```python
from build123d import *

# Parameters (mm, degrees)
SKETCH1_R              = 6.35
SKETCH1_R_2            = 3.175
BOSS_EXTRUDE1_DEPTH    = 12.7
CUT_EXTRUDE1_DEPTH     = 10.795
CUT_EXTRUDE2_START     = -29
CUT_EXTRUDE2_OUTLINE_R = 1.905
CUT_EXTRUDE2_DEPTH     = 58
SKETCH3_R              = 8.128
SKETCH3_R_2            = 6.35
BOSS_EXTRUDE2_DEPTH    = 1.27
SKETCH4_R              = 1.5875
SKETCH4_R_2            = 1.143
CUT_EXTRUDE3_DEPTH     = 31.75
SKETCH5_R              = 1.905
CUT_EXTRUDE4_DEPTH     = 7.62
SKETCH6_W              = 3.175
SKETCH6_H              = 7.353822806
CUT_EXTRUDE5_DEPTH     = 1.016
SKETCH7_R              = 4.445
CUT_EXTRUDE6_DEPTH     = 1.27


with BuildPart() as part:
    # Sketch1 → Boss-Extrude1 (new body)
    with BuildSketch(Plane.XY):
        with BuildLine():
            Line((-15.875, 228.6), (-15.875, 41.885940063))
            ThreePointArc((-15.875, 41.885940063), (-17.859739298, 27.82498979), (-23.658870968, 14.862752926))
            ThreePointArc((-23.658870968, 14.862752926), (-27.242520167, -6.203925768), (-14.890307558, -23.641538462))
            Line((-14.890307558, -23.641538462), (-4.737825132, -30.035944056))
            ThreePointArc((-4.737825132, -30.035944056), (0, -31.403636364), (4.737825132, -30.035944056))
            Line((4.737825132, -30.035944056), (14.890307558, -23.641538462))
            ThreePointArc((14.890307558, -23.641538462), (27.242520167, -6.203925768), (23.658870968, 14.862752926))
            ThreePointArc((23.658870968, 14.862752926), (17.859739298, 27.82498979), (15.875, 41.885940063))
            Line((15.875, 41.885940063), (15.875, 228.6))
            ThreePointArc((15.875, 228.6), (0, 244.475), (-15.875, 228.6))
        make_face()
        Circle(SKETCH1_R, mode=Mode.SUBTRACT)
        with Locations((0, 228.6)):
            Circle(SKETCH1_R_2, mode=Mode.SUBTRACT)
    extrude(amount=BOSS_EXTRUDE1_DEPTH)

    # Sketch2 → Cut-Extrude1 (cut)
    with BuildSketch(Plane.XY.offset(12.7)):
        with BuildLine():
            Line((-11.43, 222.25), (11.43, 222.25))
            ThreePointArc((11.43, 222.25), (13.226051224, 221.506051224), (13.97, 219.71))
            Line((13.97, 219.71), (13.97, 21.969531743))
            ThreePointArc((13.97, 21.969531743), (0, -26.035), (-13.97, 21.969531743))
            Line((-13.97, 21.969531743), (-13.97, 219.71))
            ThreePointArc((-13.97, 219.71), (-13.226051224, 221.506051224), (-11.43, 222.25))
        make_face()
    extrude(amount=-CUT_EXTRUDE1_DEPTH, mode=Mode.SUBTRACT)

    # Cut-Extrude2: read off the stored shape, not the designer's step
    # Cut-Extrude2 outline → Cut-Extrude2 (cut)
    with BuildSketch(Plane.YZ.offset(CUT_EXTRUDE2_START)):
        with Locations((0, 6.985)):
            Circle(CUT_EXTRUDE2_OUTLINE_R)
    extrude(amount=CUT_EXTRUDE2_DEPTH, mode=Mode.SUBTRACT)

    # Sketch3 → Boss-Extrude2 (add)
    with BuildSketch(Plane.XY.offset(1.905)):
        Circle(SKETCH3_R)
        Circle(SKETCH3_R_2, mode=Mode.SUBTRACT)
    extrude(amount=BOSS_EXTRUDE2_DEPTH)

    # Sketch4 → Cut-Extrude3 (cut)
    with BuildSketch(Plane.XY.offset(12.7)):
        with Locations((0, 219.71)):
            Circle(SKETCH4_R)
        with Locations((-6.35, 184.15)):
            Circle(SKETCH4_R_2)
        with Locations((6.35, 184.15)):
            Circle(SKETCH4_R_2)
        with Locations((-6.35, 69.85)):
            Circle(SKETCH4_R_2)
        with Locations((6.35, 69.85)):
            Circle(SKETCH4_R_2)
        with Locations((-16.764, 23.241)):
            Circle(SKETCH4_R_2)
        with Locations((16.764, 23.241)):
            Circle(SKETCH4_R_2)
        with Locations((0, -28.575)):
            Circle(SKETCH4_R_2)
        with Locations((-10.4775, 28.1178)):
            Circle(SKETCH4_R_2)
        with Locations((10.4775, 28.1178)):
            Circle(SKETCH4_R_2)
    extrude(amount=-CUT_EXTRUDE3_DEPTH, mode=Mode.SUBTRACT)

    # Sketch5 → Cut-Extrude4 (cut)
    with BuildSketch(Plane.XY.offset(12.7)):
        with Locations((-11.43, 228.6)):
            Circle(SKETCH5_R)
        with Locations((-9.898670365, 234.315)):
            Circle(SKETCH5_R)
        with Locations((-5.715, 238.498670365)):
            Circle(SKETCH5_R)
        with Locations((0, 240.03)):
            Circle(SKETCH5_R)
        with Locations((5.715, 238.498670365)):
            Circle(SKETCH5_R)
        with Locations((9.898670365, 234.315)):
            Circle(SKETCH5_R)
        with Locations((11.43, 228.6)):
            Circle(SKETCH5_R)
    extrude(amount=-CUT_EXTRUDE4_DEPTH, mode=Mode.SUBTRACT)

    # Sketch6 → Cut-Extrude5 (cut)
    with BuildSketch(Plane(origin=(0, 0, 0), x_dir=(-1, 0, 0), z_dir=(0, 0, -1))):
        with Locations((0, 223.386911403)):
            Rectangle(SKETCH6_W, SKETCH6_H)
    extrude(amount=-CUT_EXTRUDE5_DEPTH, mode=Mode.SUBTRACT)

    # Sketch7 → Cut-Extrude6 (cut)
    with BuildSketch(Plane(origin=(0, 0, 0), x_dir=(-1, 0, 0), z_dir=(0, 0, -1))):
        with Locations((0, 228.6)):
            Circle(SKETCH7_R)
    extrude(amount=-CUT_EXTRUDE6_DEPTH, mode=Mode.SUBTRACT)


solid = part.part
```
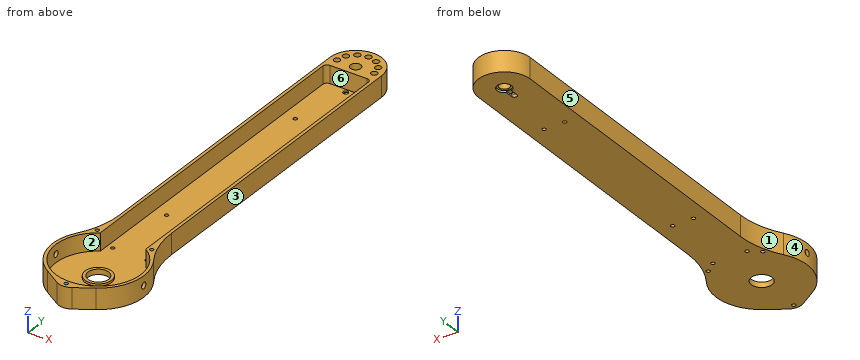
Build history of the part. All positions in model axes, mm. Face numbers are marked on the shaded views. A direction names the side the tool comes from. Round coordinates to 2 decimals unless told otherwise and drop trailing zeros. Order: outer loops, then holes, each group sorted by start corner. A loop starts at its lowest first (then second) coordinate and runs counter-clockwise, first axis right, second up. Notation, with made-up numbers: (74.5, 71) -> (123.5, 71) arc R20 cw to (123.5, 78) -> close; hole circle Ø11 at (34, 30). An arc over 180 degrees is marked (long way). Answer in a Markdown table with one row per item.
1) Which spindle directions (+Z, -Z, +X, -X, +Y, -Y) get a long thin tool onto all of the face, cutting with end or side? Do the marked faces 1, 2 and 3. Say none if no direction does.
Values:
| item | result |
|---|---|
| face 1 | +Z, -Z, -X, +Y |
| face 2 | +Z |
| face 3 | +Z, -Z, +X, +Y |
2) Band-saw the part on B-B on y = -14. Give the cut face in (x, z) (3 decimals), and give its area (3 significant figures).
Values:
| item | result |
|---|---|
| outline | (-24.179, 0) -> (24.179, 0) -> (24.179, 12.7) -> (21.95, 12.7) -> (21.95, 1.905) -> (-21.95, 1.905) -> (-21.95, 12.7) -> (-24.179, 12.7) -> close |
| area | 140 mm2 |
3) Pin check, flat tips, straight feed: P1, Ø1.4, axis at x = 10.48, y = 28.12, coming from the -Z side; P2, Ø2, axis at x = 15.5, z = 2, coming from the -Y side; P3, Ø13, axis at x = -2, y = -1.5, coming from the +Z side (3 decimals); P4, Ø2, axis at x = -3, z = 6.5, coming from the -Y side. Stop position of each tip, or through.
Values:
| item | result |
|---|---|
| P1 | through |
| P2 | y = -23.89 |
| P3 | z = 3.175 |
| P4 | y = -31.18 |
4) Band-saw the part on A-A on y = 100.5. Give the cut face in (x, z) (3 decimals).
Values:
| item | result |
|---|---|
| outline | (-15.875, 0) -> (15.875, 0) -> (15.875, 12.7) -> (13.97, 12.7) -> (13.97, 1.905) -> (-13.97, 1.905) -> (-13.97, 12.7) -> (-15.875, 12.7) -> close |
5) Wall check: L1, parallel to Y at x = 0, z = 7.25 (3 decimals); L2, parallel to X at y = 228.6, z = 9.75 (3 decimals); L3, parallel to Y at x = 12, z = 8.5. Give the ranges that are in metal, low to high.
Values:
| item | result |
|---|---|
| L1 | -31.404 to -29.718, -27.432 to -26.035, 222.25 to 225.425, 231.775 to 238.125, 241.935 to 244.475 |
| L2 | -15.875 to -13.335, -9.525 to -3.175, 3.175 to 9.525, 13.335 to 15.875 |
| L3 | -25.46 to -23.1, 222.19 to 226.78, 230.42 to 238.99 |
6) Mould opens along Y. For the marked faces 4, 5 and 6 say: released by +Y, released by -Y, zero draft, split by the parting line, or undercut.
Values:
| item | result |
|---|---|
| face 4 | split by the parting line |
| face 5 | zero draft |
| face 6 | undercut |
